```python
from build123d import *

# Parameters (mm, degrees)
BOSS_EXTRUDE1_DEPTH = 5
BOSS_EXTRUDE3_DEPTH = 33
SKETCH4_W           = 25
SKETCH4_H           = 5
BOSS_EXTRUDE4_DEPTH = 7
SKETCH5_W           = 8
SKETCH5_H           = 5
BOSS_EXTRUDE5_DEPTH = 5
SKETCH6_R           = 1.6
CUT_EXTRUDE1_DEPTH  = 5


with BuildPart() as part:
    # Sketch1 → Boss-Extrude1 (new body)
    with BuildSketch(Plane(origin=(0, 0, 0), x_dir=(1, 0, 0), z_dir=(0, 1, 0))):
        Polygon((-8.5, 10), (-8.5, -30), (-16.5, -30), (-16.5, 30), (16.5, 30), (16.5, 10), align=None)
    extrude(amount=BOSS_EXTRUDE1_DEPTH)

    # Sketch3 → Boss-Extrude3 (add)
    with BuildSketch(Plane(origin=(16.5, 0, 0), x_dir=(0, 0, -1), z_dir=(1, 0, 0))):
        Polygon((17.443375673, -2.5), (16, 0), (13.5, 0), (12.056624327, -2.5), align=None)
        Polygon((22.556624327, -2.5), (27.943375673, -2.5), (26.5, 0), (24, 0), align=None)
    extrude(amount=-BOSS_EXTRUDE3_DEPTH)

    # Sketch4 → Boss-Extrude4 (add)
    with BuildSketch(Plane.XY.offset(-10)):
        with Locations((4, 2.5)):
            Rectangle(SKETCH4_W, SKETCH4_H)
    extrude(amount=BOSS_EXTRUDE4_DEPTH)

    # Sketch5 → Boss-Extrude5 (add)
    with BuildSketch(Plane.XY.offset(30)):
        with Locations((-12.5, 2.5)):
            Rectangle(SKETCH5_W, SKETCH5_H)
    extrude(amount=BOSS_EXTRUDE5_DEPTH)

    # Sketch6 → Cut-Extrude1 (cut)
    with BuildSketch(Plane(origin=(0, 5, 0), x_dir=(1, 0, 0), z_dir=(0, 1, 0))):
        with Locations((12.5, 7)):
            Circle(SKETCH6_R)
        with Locations((-12.5, -31)):
            Circle(SKETCH6_R)
    extrude(amount=-CUT_EXTRUDE1_DEPTH, mode=Mode.SUBTRACT)


solid = part.part
```
The model under review builds one solid part; all positions refer to its coordinate system, in mm. A direction names the side the tool comes from. Give positions to 0.01 mm unless a question says otherwise; leave off trailing zeros. Write each loop counter-clockwise with the first axis right and the second up, starting at its lowest first coordinate (ties: lowest second). Pieces come first, ordered by that corner, then holes. Notation, with made-up numbers: M -26,37 L 17,37 A22 cw 17,43 Z; hole C -29.75,8 d5. An arc over 180 degrees is marked long. Write item = value, one per line. Start each with the question number.
Q1. We need section A-A (x = 12.5). State the section outline as (y, z) points.
Q2. Machinability: for faces 4 (the face through (16.5, 2, -17)), 5 (the face through (0.23, -1.23, -23.29)), 6 (the face through (-16.5, 2, 2)), 7 (the face through (4, 3, -3)), 8 (the face through (0.23, -1.23, -12.79)), which of the approach directions +Z, -Z, +X, -X, +Y, -Y give a long, thin tool a straight path to every point of the face, cutting with its end or side? Answer none if there is none.
Q3. For line 1 (Z direction, x = 12.5, y = 3.9); line 2 (X direction, y = 3.05, z = -7); line 3 (X direction, y = 2.2, z = 31), list the stretches that pass through material, from the lowest coordinate up.
Q4. We need section D-D (x = -3). State the section outline as (y, z) points, plus the area to 3 significant figures.
Q5. Mouldability with a two-part tool opening along Z and no side actions: class faces 1 (the face through (0, 0, -28)), 2 (the face through (-14.1, 2.54, 30.93)), 3 (the face through (0, 2, -30)) as released by +Z, released by -Z, zero draft, split by the parting line, or undercut.
Q6. Clearance check with flat-ended pins moving along their axes: pin 1 (4 mm diameter, centred on x = 8, y = 3, fed in from +Z); pin 2 (4 mm diameter, centred on x = 1, z = -19, fed in from -Y); pin 3 (1.5 mm diameter, centred on x = 2.5, y = -1.5, fed in from +Z); pin 4 (1.5 mm diameter, centred on y = 1.5, z = 3, fed in from +X). State where each tip first meets the part, or that it passes through.
Q7. We need section C-C (y = 3). State the section outline as (x, z) points, plus the area to 3 significant figures.
Q8. We need section B-B (z = 31). State the section outline as (x, y) points.
Result set:
q1.outline = M -2.5,-27.94 L 0,-26.5 L 0,-30 L 5,-30 L 5,-8.6 L 0,-8.6 L 0,-13.5 L -2.5,-12.06 L -2.5,-17.44 L 0,-16 L 0,-24 L -2.5,-22.56 Z; M 0,-5.4 L 5,-5.4 L 5,-3 L 0,-3 Z
q2.face_4 = +Z, -Z, +X, +Y, -Y
q2.face_5 = +X, -X
q2.face_6 = +Z, -Z, -X, +Y, -Y
q2.face_7 = +Z, +X, +Y, -Y
q2.face_8 = +Z, +X, -X
q3.line_1 = -30 to -8.6, -5.4 to -3
q3.line_2 = -16.5 to 10.9, 14.1 to 16.5
q3.line_3 = -16.5 to -14.1, -10.9 to -8.5
q4.outline = M -2.5,-27.94 L 0,-26.5 L 0,-30 L 5,-30 L 5,-3 L 0,-3 L 0,-13.5 L -2.5,-12.06 L -2.5,-17.44 L 0,-16 L 0,-24 L -2.5,-22.56 Z
q4.area = 155 mm2
q5.face_1 = zero draft
q5.face_2 = undercut
q5.face_3 = released by -Z
q6.pin_1 = -3
q6.pin_2 = -2.5
q6.pin_3 = -12.2
q6.pin_4 = -8.5
q7.outline = M -16.5,-30 L 16.5,-30 L 16.5,-3 L -8.5,-3 L -8.5,35 L -16.5,35 Z; hole C -12.5,31 d3.2; hole C 12.5,-7 d3.2
q7.area = 1,180 mm2
q8.outline = M -16.5,0 L -14.1,0 L -14.1,5 L -16.5,5 Z; M -10.9,0 L -8.5,0 L -8.5,5 L -10.9,5 Z
